For this review, take the finished solid that the model builds, in its own axes (mm). Face numbers are marked on the shaded views. A direction names the side the tool comes from. Give positions to 0.01 mm unless a question says otherwise; leave off trailing zeros. Write each loop counter-clockwise with the first axis right and the second up, starting at its lowest first coordinate (ties: lowest second). Pieces come first, ordered by that corner, then holes. Notation, with made-up numbers: M -2.75,25 L 45.25,25 A30 cw 45.25,49 Z; hole C 20.25,42.25 d3. An arc over 180 degrees is marked long. Use one line per item in the form item = value. Start each with the question number.
Q1. Mouldability with a two-part tool opening along Y and no side actions: class the marked faces 1, 2 and 3 as released by +Y, released by -Y, zero draft, split by the parting line, or undercut.
Q2. Consider section B-B on x = -6.75. Write out the cut boundary in (y, z), and give its area (3 significant figures).
Q3. For probe 1 along Z at (x, y) = (0, 7.5); probe 2 along Y at (x, z) = (5.5, -5.5); probe 3 along Z at (x, y) = (0, 3), list the stretches that pass through material, from the lowest coordinate up. Write a range as [from, to].
Q4. Consider section D-D on x = 0.5. Write out the cut boundary in (y, z), and give its area (3 significant figures).
Q5. Consider section A-A on z = 0. Write out the cut boundary in (x, y), and give its area (3 significant figures).
Q6. Consider section C-C on y = 12.5. Write out the cut boundary in (x, z), and give its area (3 significant figures).
Q7. Clearance check with flat-ended pins moving along their axes: pin 1 Ø3 at (y, z) = (2.5, 0) entering from -X; pin 2 Ø5 at (x, y) = (2.5, 6) entering from -Z; pin 3 Ø1.5 at (y, z) = (13, -1) entering from -X. State where each tip first meets the part, or that it passes through.
Q8. Tool access review of the marked faces 4, 5 and 6: name each direction out of +Z, -Z, +X, -X, +Y, -Y from which nothing blocks a thin tool from reaching the whole face with its end or side.
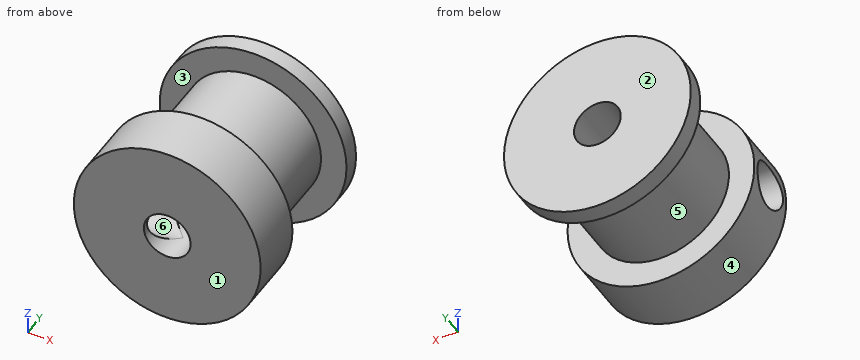
```python
from build123d import *

# Parameters (mm, degrees)
CROQUIS1_R              = 8
CROQUIS1_R_2            = 2
SALIENTE_EXTRUIR1_DEPTH = 5
CROQUIS1_3_R            = 5.82
CROQUIS1_3_R_2          = 2
SALIENTE_EXTRUIR2_DEPTH = 13.5
CROQUIS2_R              = 8
CROQUIS2_R_2            = 2
SALIENTE_EXTRUIR7_DEPTH = 1.5
CORTAR_EXTRUIR1_REACH   = 10
CROQUIS3_R              = 2


with BuildPart() as part:
    # Croquis1 → Saliente-Extruir1 (new body)
    with BuildSketch(Plane(origin=(0, 0, 0), x_dir=(1, 0, 0), z_dir=(0, 1, 0))):
        Circle(CROQUIS1_R)
        Circle(CROQUIS1_R_2, mode=Mode.SUBTRACT)
    extrude(amount=SALIENTE_EXTRUIR1_DEPTH)

    # Croquis1_3 → Saliente-Extruir2 (add)
    with BuildSketch(Plane(origin=(0, 0, 0), x_dir=(1, 0, 0), z_dir=(0, 1, 0))):
        Circle(CROQUIS1_3_R)
        Circle(CROQUIS1_3_R_2, mode=Mode.SUBTRACT)
    extrude(amount=SALIENTE_EXTRUIR2_DEPTH)

    # Croquis2 → Saliente-Extruir7 (add)
    with BuildSketch(Plane(origin=(0, 13.5, 0), x_dir=(1, 0, 0), z_dir=(0, 1, 0))):
        Circle(CROQUIS2_R)
        Circle(CROQUIS2_R_2, mode=Mode.SUBTRACT)
    extrude(amount=SALIENTE_EXTRUIR7_DEPTH)

    # Croquis3 → Cortar-Extruir1 (cut, up to next)
    with BuildSketch(Plane(origin=(0, 0, 0), x_dir=(0, 0, -1), z_dir=(1, 0, 0)), mode=Mode.PRIVATE) as cortar_extruir1_sk1:
        with Locations((0, 2.5)):
            Circle(CROQUIS3_R)
    cortar_extruir1_tool1 = extrude(cortar_extruir1_sk1.sketch, amount=-CORTAR_EXTRUIR1_REACH, mode=Mode.PRIVATE) & part.part
    add(cortar_extruir1_tool1.solids().sort_by_distance((0, 2.5, 0))[0], mode=Mode.SUBTRACT)


solid = part.part
```
Working result:
q1.face_1 = released by -Y
q1.face_2 = released by +Y
q1.face_3 = undercut
q2.outline = M 0,-4.29 L 5,-4.29 L 5,4.29 L 0,4.29 Z; M 13.5,-4.29 L 15,-4.29 L 15,4.29 L 13.5,4.29 Z; hole C 2.5,0 d4
q2.area = 43.3 mm²
q3.probe_1 = [-5.82, -2], [2, 5.82]
q3.probe_2 = [0, 5], [13.5, 15]
q3.probe_3 = [-8, -2], [2, 8]
q4.outline = M 0,-7.98 L 5,-7.98 L 5,-5.8 L 13.5,-5.8 L 13.5,-7.98 L 15,-7.98 L 15,-1.94 L 0,-1.94 Z; M 0,1.94 L 15,1.94 L 15,7.98 L 13.5,7.98 L 13.5,5.8 L 5,5.8 L 5,7.98 L 0,7.98 Z
q4.area = 144 mm²
q5.outline = M -8,0 L -2,0 L -2,0.5 L -8,0.5 Z; M -8,4.5 L -2,4.5 L -2,15 L -8,15 L -8,13.5 L -5.82,13.5 L -5.82,5 L -8,5 Z; M 2,0 L 8,0 L 8,5 L 5.82,5 L 5.82,13.5 L 8,13.5 L 8,15 L 2,15 Z
q5.area = 119 mm²
q6.outline = C 0,0 d11.64; hole C 0,0 d4
q6.area = 93.8 mm²
q7.pin_1 = 1.32
q7.pin_2 = -8
q7.pin_3 = -7.99
q8.face_4 = +Y, -Y
q8.face_5 = none
q8.face_6 = -X
